Design review of the part built by this model. Coordinates are the model's own, in mm. Face numbers are marked on the shaded views. Round coordinates to 2 decimals unless told otherwise and drop trailing zeros. Loops run counter-clockwise (first coordinate to the right, second up) from the corner with the lowest first, then second, coordinate; pieces in that order, holes last. Notation, with made-up numbers: (69.5, 43) -> (120.5, 43) arc R6 ccw to (120.5, 52) -> close; hole circle Ø10 at (24.25, 80.25). An arc over 180 degrees is marked (long way). Answer as CSV lines item,"result". Start each with the question number.
(1) To check wall thickness, follow line 1 (Y direction, x = 79.2, z = 11); line 2 (Y direction, x = -53.5, z = 26.25). State the ranges of each line that lie inside material, in increasing order. Write a range as from..to.
(2) Take a section at A-A, the plane x = 49. Write out the cut boundary in (y, z), and give its area (3 significant figures).
(3) Draft analysis for pull direction Y (two halves, no side actions). For the marked faces 1, 2 and 3, state which applies: +Y half, -Y half, draft (parallel to the pull), parting line (faces both ways), or undercut.
(4) For P1, Ø5, axis at x = -79.2, y = 79.2, coming from the -Z side; P2, Ø4, axis at x = -84.5, z = 9.5, coming from the +Y side; P3, Ø7.5, axis at x = 81.5, y = 79, coming from the +Z side, all flat-tipped, find the tip position at first contact; note any pin that passes through.
from build123d import *

# Parameters (mm, degrees)
SKETCH2_W                = 200
SKETCH2_H                = 200
BOSS_EXTRUDE1_DEPTH      = 30
FILLET1_R                = 20
CUT_EXTRUDE1_DEPTH       = 3
CUT_EXTRUDE2_DEPTH       = 144.975692393
SKETCH6_W                = 15
SKETCH6_H                = 15
BOSS_EXTRUDE4_DEPTH      = 15
FILLET2_R                = 5
F_4_0_4_DIAMETER_HOLE1_D = 4
CUT_EXTRUDE3_START       = -6.6
CUT_EXTRUDE3_DEPTH       = 6.6
CUT_EXTRUDE4_REACH       = 227.61
SKETCH11_R               = 1.5
SKETCH15_R               = 1
CUT_EXTRUDE5_DEPTH       = 217.094053597
CUT_EXTRUDE7_DEPTH       = 9.8
FILLET3_R                = 1


with BuildPart() as part:
    # Sketch2 → Boss-Extrude1 (new body)
    with BuildSketch(Plane.XY):
        Rectangle(SKETCH2_W, SKETCH2_H)
    extrude(amount=BOSS_EXTRUDE1_DEPTH)

    # Fillet1
    fillet1_edges = [part.edges().sort_by_distance(p)[0] for p in [
        (100, -100, 15),
        (-100, -100, 15),
        (-100, 100, 15),
        (100, 100, 15),
    ]]
    fillet(fillet1_edges, radius=FILLET1_R)

    # Sketch3 → Cut-Extrude1 (cut)
    with BuildSketch(Plane.XY.offset(30)):
        with BuildLine():
            Line((-90, 80), (-90, -80))
            ThreePointArc((-90, -80), (-87.071067812, -87.071067812), (-80, -90))
            Line((-80, -90), (80, -90))
            ThreePointArc((80, -90), (87.071067812, -87.071067812), (90, -80))
            Line((90, -80), (90, 80))
            ThreePointArc((90, 80), (87.071067812, 87.071067812), (80, 90))
            Line((80, 90), (-80, 90))
            ThreePointArc((-80, 90), (-87.071067812, 87.071067812), (-90, 80))
        make_face()
    extrude(amount=-CUT_EXTRUDE1_DEPTH, mode=Mode.SUBTRACT)

    # Sketch4 → Cut-Extrude2 (cut, through all)
    with BuildSketch(Plane.XY.offset(27)):
        with BuildLine():
            Line((-89.2, 80), (-89.2, -80))
            ThreePointArc((-89.2, -80), (-86.505382387, -86.505382387), (-80, -89.2))
            Line((-80, -89.2), (80, -89.2))
            ThreePointArc((80, -89.2), (86.505382387, -86.505382387), (89.2, -80))
            Line((89.2, -80), (89.2, 80))
            ThreePointArc((89.2, 80), (86.505382387, 86.505382387), (80, 89.2))
            Line((80, 89.2), (-80, 89.2))
            ThreePointArc((-80, 89.2), (-86.505382387, 86.505382387), (-89.2, 80))
        make_face()
    extrude(amount=-CUT_EXTRUDE2_DEPTH, mode=Mode.SUBTRACT)

    # Sketch6 → Boss-Extrude4 (add)
    with BuildSketch(Plane(origin=(0, 0, 0), x_dir=(-1, 0, 0), z_dir=(0, 0, -1))):
        with Locations((-81.7, -81.7)):
            Rectangle(SKETCH6_W, SKETCH6_H)
        with Locations((-81.7, 81.7)):
            Rectangle(SKETCH6_W, SKETCH6_H)
        with Locations((81.7, 81.7)):
            Rectangle(SKETCH6_W, SKETCH6_H)
        with Locations((81.7, -81.7)):
            Rectangle(SKETCH6_W, SKETCH6_H)
    extrude(amount=-BOSS_EXTRUDE4_DEPTH)

    # Fillet2
    fillet2_edges = [part.edges().sort_by_distance(p)[0] for p in [
        (74.2, 74.2, 7.5),
        (-74.2, 74.2, 7.5),
        (-74.2, -74.2, 7.5),
        (74.2, -74.2, 7.5),
    ]]
    fillet(fillet2_edges, radius=FILLET2_R)

    # Ø4.0 (4) Diameter Hole1 (through all)
    with Locations(Plane(origin=(0, 0, 0), x_dir=(-1, 0, 0), z_dir=(0, 0, -1))):
        with Locations((-79.2, 79.2), (79.2, 79.2), (-79.2, -79.2), (79.2, -79.2)):
            Hole(F_4_0_4_DIAMETER_HOLE1_D / 2)

    # Sketch10 → Cut-Extrude3 (cut)
    with BuildSketch(Plane(origin=(0, 0, 0), x_dir=(-1, 0, 0), z_dir=(0, 0, -1)).offset(CUT_EXTRUDE3_START)):
        with BuildLine():
            Line((89.2, -80), (89.2, 80))
            ThreePointArc((89.2, 80), (86.505382387, 86.505382387), (80, 89.2))
            Line((80, 89.2), (-80, 89.2))
            ThreePointArc((-80, 89.2), (-86.505382387, 86.505382387), (-89.2, 80))
            Line((-89.2, 80), (-89.2, -80))
            ThreePointArc((-89.2, -80), (-86.505382387, -86.505382387), (-80, -89.2))
            Line((-80, -89.2), (80, -89.2))
            ThreePointArc((80, -89.2), (86.505382387, -86.505382387), (89.2, -80))
        make_face()
    extrude(amount=CUT_EXTRUDE3_DEPTH, mode=Mode.SUBTRACT)

    # Sketch11 → Cut-Extrude4 (cut, up to next)
    with BuildSketch(Plane(origin=(0, 100, 0), x_dir=(1, 0, 0), z_dir=(0, 1, 0)), mode=Mode.PRIVATE) as cut_extrude4_sk1:
        with Locations(Location((-68.95500318, -14.324851484, 0), (0, 0, 270))):
            Circle(SKETCH11_R)
    cut_extrude4_tool1 = extrude(cut_extrude4_sk1.sketch, amount=-CUT_EXTRUDE4_REACH, mode=Mode.PRIVATE) & part.part
    add(cut_extrude4_tool1.solids().sort_by_distance((-68.955003, 100, 14.324851))[0], mode=Mode.SUBTRACT)

    # Sketch15 → Cut-Extrude5 (cut, through all)
    with BuildSketch(Plane(origin=(-89.2, 0, 0), x_dir=(0, 0, -1), z_dir=(1, 0, 0))):
        with Locations((-9.506010444, -49.23845191)):
            Circle(SKETCH15_R)
        with BuildLine():
            Line((-9.226010444, -59.688663791), (-9.786010444, -59.688663791))
            ThreePointArc((-9.786010444, -59.688663791), (-11.05880265, -60.215871585), (-11.586010444, -61.488663791))
            Line((-11.586010444, -61.488663791), (-11.586010444, -67.838663791))
            ThreePointArc((-11.586010444, -67.838663791), (-11.05880265, -69.111455997), (-9.786010444, -69.638663791))
            Line((-9.786010444, -69.638663791), (-9.226010444, -69.638663791))
            ThreePointArc((-9.226010444, -69.638663791), (-7.953218238, -69.111455997), (-7.426010444, -67.838663791))
            Line((-7.426010444, -67.838663791), (-7.426010444, -61.488663791))
            ThreePointArc((-7.426010444, -61.488663791), (-7.953218238, -60.215871585), (-9.226010444, -59.688663791))
        make_face()
    extrude(amount=-CUT_EXTRUDE5_DEPTH, mode=Mode.SUBTRACT)

    # Sketch17 → Cut-Extrude7 (cut)
    with BuildSketch(Plane.ZY.offset(100)):
        with BuildLine():
            Line((20.850135553, -38.354466572), (7.5, -38.354466572))
            ThreePointArc((7.5, -38.354466572), (3.964466094, -39.818932666), (2.5, -43.354466572))
            Line((2.5, -43.354466572), (2.5, -72.5))
            ThreePointArc((2.5, -72.5), (3.964466094, -76.035533906), (7.5, -77.5))
            Line((7.5, -77.5), (20.850135553, -77.5))
            ThreePointArc((20.850135553, -77.5), (24.385669459, -76.035533906), (25.850135553, -72.5))
            Line((25.850135553, -72.5), (25.850135553, -43.354466572))
            ThreePointArc((25.850135553, -43.354466572), (24.385669459, -39.818932666), (20.850135553, -38.354466572))
        make_face()
    extrude(amount=-CUT_EXTRUDE7_DEPTH, mode=Mode.SUBTRACT)

    # Fillet3
    fillet3_edges = [part.edges().sort_by_distance(p)[0] for p in [
        (-100, -39.818932666, 3.964466094),
        (-100, -57.927233286, 2.5),
        (-100, -76.035533906, 3.964466094),
        (-100, -77.5, 14.175067777),
        (-100, -76.035533906, 24.385669459),
        (-100, -57.927233286, 25.850135553),
        (-100, -39.818932666, 24.385669459),
        (-100, -38.354466572, 14.175067777),
        (-90.2, -39.818932666, 3.964466094),
        (-90.2, -38.354466572, 14.175067777),
        (-90.2, -39.818932666, 24.385669459),
        (-90.2, -57.927233286, 25.850135553),
        (-90.2, -76.035533906, 24.385669459),
        (-90.2, -77.5, 14.175067777),
        (-90.2, -76.035533906, 3.964466094),
        (-90.2, -57.927233286, 2.5),
    ]]
    fillet(fillet3_edges, radius=FILLET3_R)


solid = part.part
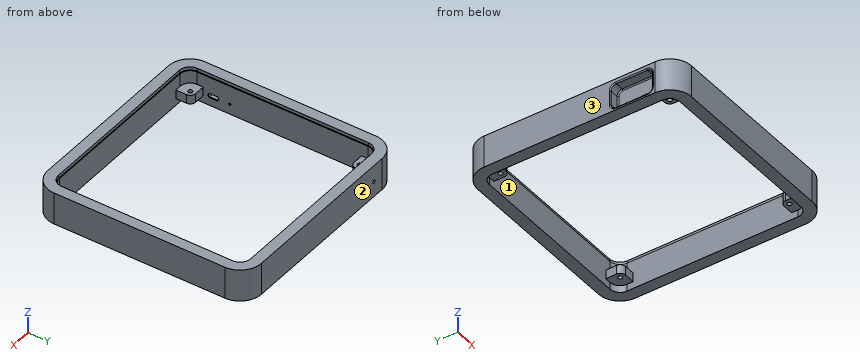
The answers:
1,line 1,"-100..-81.2, -77.2..-74.2, 74.2..77.2, 81.2..100"
1,line 2,"-100..-89.2, 89.2..100"
2,outline,"(-100, 0) -> (-89.2, 0) -> (-89.2, 27) -> (-90, 27) -> (-90, 30) -> (-100, 30) -> close; (89.2, 0) -> (100, 0) -> (100, 30) -> (90, 30) -> (90, 27) -> (89.2, 27) -> close"
2,area,"643 mm²"
3,face 1,"undercut"
3,face 2,"+Y half"
3,face 3,"draft"
4,P1,"z = 6.6"
4,P2,"y = 99.84"
4,P3,"z = 15"
